from build123d import *

# Parameters (mm, degrees)
SKETCH1_R           = 10.1
BOSS_EXTRUDE1_DEPTH = 11.9
SKETCH1_4_R         = 1.6
CUT_EXTRUDE1_DEPTH  = 6
CHAMFER1_SIZE       = 1


with BuildPart() as part:
    # Sketch1 → Boss-Extrude1 (new body)
    with BuildSketch(Plane(origin=(0, 0, 0), x_dir=(1, 0, 0), z_dir=(0, 1, 0))):
        with Locations(Location((0, 0, 0), (0, 0, 270))):
            Circle(SKETCH1_R)
    extrude(amount=BOSS_EXTRUDE1_DEPTH)

    # Sketch1_4 → Cut-Extrude1 (cut)
    with BuildSketch(Plane(origin=(0, 0, 0), x_dir=(1, 0, 0), z_dir=(0, 1, 0))):
        with Locations(Location((0, 0, 0), (0, 0, 270))):
            Circle(SKETCH1_4_R)
    extrude(amount=CUT_EXTRUDE1_DEPTH, mode=Mode.SUBTRACT)

    # Chamfer1
    chamfer1_edges = [part.edges().sort_by_distance(p)[0] for p in [
        (0, 0, -10.1),
        (0, 11.9, -10.1),
    ]]
    chamfer(chamfer1_edges, length=CHAMFER1_SIZE)


solid = part.part
Work out the finished part from the listing and answer in its coordinate system (mm). A direction names the side the tool comes from. Coordinates: 2 decimals unless noted, no trailing zeros. Write each loop counter-clockwise with the first axis right and the second up, starting at its lowest first coordinate (ties: lowest second). Pieces come first, ordered by that corner, then holes. Notation, with made-up numbers: M -12.5,89 L 28.5,89 A28 cw 28.5,114 Z; hole C -38.5,10 d11. An arc over 180 degrees is marked long. Use one line per item in the form item = value. Start each with the question number.
1. The part is cut by section D-D (y = 9.25). Give the vertices of the cut face in (x, z), plus the area to 3 significant figures.
2. The mould has two halves that part along X. Classify faces 1 (the face through (0, 11.9, 0)), 2 (the face through (-6.146, 5.881, -8.015)), 3 (the face through (-0.97, 2.96, -1.27)): released by +X, released by -X, zero draft, split by the parting line, or undercut.
3. A tool of negligible diameter and unlimited length cuts with its end or side. For faces 4 (the face through (0, 0, 2)), 5 (the face through (0, 6, 0)), from which of +Z, -Z, +X, -X, +Y, -Y can it reach the whole face along a straight path? Write none if from no direction.
4. The part is cut by section B-B (x = 0). Give the vertices of the cut face in (y, z), plus the area to 3 significant figures.
5. Straight lines are drawn through the part: probe 1 along X at (y, z) = (1.4, 0); probe 2 along Z at (x, y) = (-7.75, 7.5); probe 3 along Z at (x, y) = (-1.5, 8.75). For each, find the intervals that lie inside material, in ascending order. Write a range as from..to.
6. The part is cut by section C-C (y = 5.5). Give the vertices of the cut face in (x, z).
7. Each of these flat-tipped pins is pushed along its axis until it touches: P1, Ø1.9, axis at x = 0, z = 0, coming from the -Y side; P2, Ø2, axis at y = 4, z = 7, coming from the -X side; P3, Ø2, axis at y = 9.5, z = -4, coming from the +X side. Where does it stop, or does it pass through?
8. The part is cut by section A-A (z = 0). Give the vertices of the cut face in (x, y), plus the area to 3 significant figures.
Evaluation:
q1.outline = C 0,0 d20.2
q1.area = 320 mm^2
q2.face_1 = zero draft
q2.face_2 = split by the parting line
q2.face_3 = undercut
q3.face_4 = +Z, -Z, +X, -X, -Y
q3.face_5 = -Y
q4.outline = M 0,-9.1 L 1,-10.1 L 10.9,-10.1 L 11.9,-9.1 L 11.9,9.1 L 10.9,10.1 L 1,10.1 L 0,9.1 L 0,1.6 L 6,1.6 L 6,-1.6 L 0,-1.6 Z
q4.area = 219 mm^2
q5.probe_1 = -10.1..-1.6, 1.6..10.1
q5.probe_2 = -6.48..6.48
q5.probe_3 = -9.99..9.99
q6.outline = C 0,0 d20.2; hole C 0,0 d3.2
q7.P1 = 6
q7.P2 = -8.12
q7.P3 = 9.64
q8.outline = M -10.1,1 L -9.1,0 L -1.6,0 L -1.6,6 L 1.6,6 L 1.6,0 L 9.1,0 L 10.1,1 L 10.1,10.9 L 9.1,11.9 L -9.1,11.9 L -10.1,10.9 Z
q8.area = 219 mm^2
